```python
from build123d import *

# Parameters (mm, degrees)
F0_W     = 150
F0_H     = 152.5
F0_R     = 4
F1_DEPTH = 10
F2_R     = 5
F4_D     = 5


with BuildPart() as f1:
    # F0 (on Front) → F1 (new body)
    with BuildSketch(Plane.XZ):
        with Locations((0, -36.25)):
            Rectangle(F0_W, F0_H)
        with Locations((-62.5, -32.5)):
            Circle(F0_R, mode=Mode.SUBTRACT)
        with Locations((-62.5, 32.5)):
            Circle(F0_R, mode=Mode.SUBTRACT)
        with BuildLine():
            Line((-40, 30), (40, 30))
            ThreePointArc((40, 30), (43.5355339059, 28.5355339059), (45, 25))
            Line((45, 25), (45, -25))
            ThreePointArc((45, -25), (43.5355339059, -28.5355339059), (40, -30))
            Line((40, -30), (-40, -30))
            ThreePointArc((-40, -30), (-43.5355339059, -28.5355339059), (-45, -25))
            Line((-45, -25), (-45, 25))
            ThreePointArc((-45, 25), (-43.5355339059, 28.5355339059), (-40, 30))
        make_face(mode=Mode.SUBTRACT)
        with Locations((62.5, -32.5)):
            Circle(F0_R, mode=Mode.SUBTRACT)
        with Locations((62.5, 32.5)):
            Circle(F0_R, mode=Mode.SUBTRACT)
    extrude(amount=F1_DEPTH)

    # F2
    f2_edges = [f1.edges().sort_by_distance(p)[0] for p in [
        (-75, -5, 40),
        (75, -5, 40),
    ]]
    fillet(f2_edges, radius=F2_R)

    # F4 (through all)
    with Locations(Plane.XZ.offset(10)):
        with Locations((65, -87.5), (-65, -87.5)):
            Hole(F4_D / 2)


solid = f1.part
```
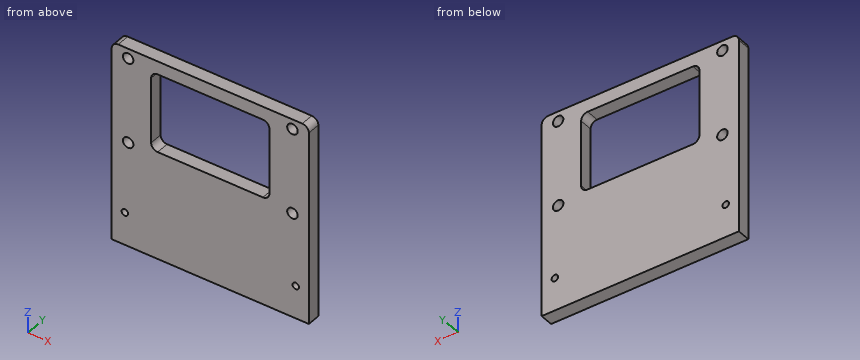
Geometry: final body of the model. Coordinates: model frame, mm. Round coordinates to 2 decimals unless told otherwise and drop trailing zeros. Write each loop counter-clockwise with the first axis right and the second up, starting at its lowest first coordinate (ties: lowest second). Pieces come first, ordered by that corner, then holes. Notation, with made-up numbers: (-23, 66.25) -> (16, 66.25) arc R14 cw to (16, 70.25) -> close; hole circle Ø4 at (12.25, 66.25). An arc over 180 degrees is marked (long way). Use CSV: the item, a comma, the result in double quotes. Start each with the question number.
Q1. Section B-B (x = -17). Return loops of the section in (y, z).
Q2. First-contact query: pin 1 Ø6.5 at (x, z) = (62.5, -32.5) entering from -Y. Flat tip, straight axial feed; report the tip coordinate or a pass-through.
Q3. Section C-C (y = -7.25). Return loops of the section in (x, z).
Q4. Section D-D (z = -19). Return loops of the section in (x, y), plus the area to 3 significant figures.
Q5. Line query: L1, parallel to X at y = -3.25, z = 10.5; L2, parallel to Z at x = 60.5, y = -5; L3, parallel to Z at x = -65, y = -4.75. Output: solid intervals per line, ascending.
Q6. Section A-A (z = 32.5). Return loops of the section in (x, y), plus the area to 3 significant figures.
Result sheet:
1,outline,"(-10, -112.5) -> (0, -112.5) -> (0, -30) -> (-10, -30) -> close; (-10, 30) -> (0, 30) -> (0, 40) -> (-10, 40) -> close"
2,pin 1,"through"
3,outline,"(-75, -112.5) -> (75, -112.5) -> (75, 35) arc R5 ccw to (70, 40) -> (-70, 40) arc R5 ccw to (-75, 35) -> close; hole circle Ø5 at (-65, -87.5); hole circle Ø8 at (-62.5, -32.5); hole circle Ø8 at (-62.5, 32.5); hole (-45, -25) arc R5 ccw to (-40, -30) -> (40, -30) arc R5 ccw to (45, -25) -> (45, 25) arc R5 ccw to (40, 30) -> (-40, 30) arc R5 ccw to (-45, 25) -> close; hole circle Ø8 at (62.5, -32.5); hole circle Ø8 at (62.5, 32.5); hole circle Ø5 at (65, -87.5)"
4,outline,"(-75, -10) -> (-45, -10) -> (-45, 0) -> (-75, 0) -> close; (45, -10) -> (75, -10) -> (75, 0) -> (45, 0) -> close"
4,area,"600 mm²"
5,L1,"-75 to -45, 45 to 75"
5,L2,"-112.5 to -35.96, -29.04 to 29.04, 35.96 to 40"
5,L3,"-112.5 to -90, -85 to -35.62, -29.38 to 29.38, 35.62 to 40"
6,outline,"(-75, -10) -> (-66.5, -10) -> (-66.5, 0) -> (-75, 0) -> close; (-58.5, -10) -> (58.5, -10) -> (58.5, 0) -> (-58.5, 0) -> close; (66.5, -10) -> (75, -10) -> (75, 0) -> (66.5, 0) -> close"
6,area,"1,340 mm²"
